```python
from build123d import *

# Parameters (mm, degrees)
SKETCH1_W           = 100
SKETCH1_H           = 80
BOSS_EXTRUDE1_DEPTH = 3.175
SKETCH3_W           = 100.17
SKETCH3_H           = 80.17
SKETCH3_W_2         = 87.47
SKETCH3_H_2         = 67.47
CUT_EXTRUDE2_DEPTH  = 10
SKETCH4_R           = 1.415
CUT_EXTRUDE3_DEPTH  = 10
SKETCH2_W           = 8.33
SKETCH2_H           = 21.08
CUT_EXTRUDE4_DEPTH  = 10


with BuildPart() as part:
    # Sketch1 → Boss-Extrude1 (new body)
    with BuildSketch(Plane.XY):
        Rectangle(SKETCH1_W, SKETCH1_H)
    extrude(amount=BOSS_EXTRUDE1_DEPTH)

    # Sketch3 → Cut-Extrude2 (cut)
    with BuildSketch(Plane.XY.offset(3.175)):
        Rectangle(SKETCH3_W, SKETCH3_H)
        Rectangle(SKETCH3_W_2, SKETCH3_H_2, mode=Mode.SUBTRACT)
    extrude(amount=-CUT_EXTRUDE2_DEPTH, mode=Mode.SUBTRACT)

    # Sketch4 → Cut-Extrude3 (cut)
    with BuildSketch(Plane.XY.offset(3.175)):
        with Locations((-40.553019485, 30.553019485)):
            Circle(SKETCH4_R)
        with Locations((40.553019485, 30.553019485)):
            Circle(SKETCH4_R)
        with Locations((40.553019485, -30.553019485)):
            Circle(SKETCH4_R)
        with Locations((-40.553019485, -30.553019485)):
            Circle(SKETCH4_R)
    extrude(amount=-CUT_EXTRUDE3_DEPTH, mode=Mode.SUBTRACT)

    # Sketch2 → Cut-Extrude4 (cut)
    with BuildSketch(Plane.XY.offset(3.175)):
        with Locations((-20.25, 14.675)):
            Rectangle(SKETCH2_W, SKETCH2_H)
        with Locations((20.25, 14.675)):
            Rectangle(SKETCH2_W, SKETCH2_H)
        with Locations((-20.25, -14.675)):
            Rectangle(SKETCH2_W, SKETCH2_H)
        with Locations((20.25, -14.675)):
            Rectangle(SKETCH2_W, SKETCH2_H)
    extrude(amount=-CUT_EXTRUDE4_DEPTH, mode=Mode.SUBTRACT)


solid = part.part
```
Source: CAD feature listing. Evaluate the final solid. Frame: model axes, mm. A direction names the side the tool comes from. Give positions to 0.01 mm unless a question says otherwise; leave off trailing zeros. Order: outer loops, then holes, each group sorted by start corner. A loop starts at its lowest first (then second) coordinate and runs counter-clockwise, first axis right, second up. Notation, with made-up numbers: (15.5, 49) -> (53.5, 49) arc R22 ccw to (53.5, 68) -> close; hole circle Ø7 at (16.25, 64.5). An arc over 180 degrees is marked (long way). Use a Markdown table: item, result.
Q1. First-contact query: P1, Ø1.7, axis at x = 40.55, y = -30.55, coming from the +Z side. Flat tip, straight axial feed; report the tip coordinate or a pass-through.
A:
| item | result |
|---|---|
| P1 | through |
Q2. Section C-C (z = 0.85). State how many separate pieces and enclosed holes the cut face has, and give its area (3 significant figures).
A:
| item | result |
|---|---|
| separate pieces | 1 |
| enclosed holes | 8 |
| area | 5,170 mm^2 |
Q3. Access query for faces 1 (the face through (-16.085, 15, 2)), 2 (the face through (-1, 0, 3.175)). Directions: +Z, -Z, +X, -X, +Y, -Y. A direction counts if a zero-diameter tool reaches every point of the face in a straight line with its end or side. Return the directions, or none.
A:
| item | result |
|---|---|
| face 1 | +Z, -Z |
| face 2 | +Z, +X, -X, +Y, -Y |
Q4. Material intervals for line 1 (X direction, y = -10, z = 1.65) (3 decimals); line 2 (Y direction, x = -22, z = 2.1) (3 decimals), sorted ascending. Write a range as [from, to].
A:
| item | result |
|---|---|
| line 1 | [-43.735, -24.415], [-16.085, 16.085], [24.415, 43.735] |
| line 2 | [-33.735, -25.215], [-4.135, 4.135], [25.215, 33.735] |
Q5. Pull-direction query (X, two-part tool) for faces 3 (the face through (-1, 33.735, 2)), 4 (the face through (-16.085, -15, 2)), 5 (the face through (43.735, 0, 2)); classes: +X half, -X half, draft (parallel to the pull), parting line (faces both ways), or undercut.
A:
| item | result |
|---|---|
| face 3 | draft |
| face 4 | undercut |
| face 5 | +X half |
Q6. Section A-A (y = -8). Return the cut outline in (x, z) (3 decimals), and give its area (3 significant figures).
A:
| item | result |
|---|---|
| outline | (-43.735, 0) -> (-24.415, 0) -> (-24.415, 3.175) -> (-43.735, 3.175) -> close; (-16.085, 0) -> (16.085, 0) -> (16.085, 3.175) -> (-16.085, 3.175) -> close; (24.415, 0) -> (43.735, 0) -> (43.735, 3.175) -> (24.415, 3.175) -> close |
| area | 225 mm^2 |
Q7. Section B-B (x = 22.5). Return the cut outline in (y, z) (3 decimals), and give its area (3 significant figures).
A:
| item | result |
|---|---|
| outline | (-33.735, 0) -> (-25.215, 0) -> (-25.215, 3.175) -> (-33.735, 3.175) -> close; (-4.135, 0) -> (4.135, 0) -> (4.135, 3.175) -> (-4.135, 3.175) -> close; (25.215, 0) -> (33.735, 0) -> (33.735, 3.175) -> (25.215, 3.175) -> close |
| area | 80.4 mm^2 |
